Read the model definition and answer for the solid it produces. Units are mm, in the model's axes. A direction names the side the tool comes from. Coordinates: 2 decimals unless noted, no trailing zeros. Write each loop counter-clockwise with the first axis right and the second up, starting at its lowest first coordinate (ties: lowest second). Pieces come first, ordered by that corner, then holes. Notation, with made-up numbers: (15.25, 36.5) - (36.25, 36.5) arc R35 ccw to (36.25, 69.5) - close; hole circle Ø2 at (35, 27.5). An arc over 180 degrees is marked (long way). Use a Markdown table: item, result.
Autodesk Inventor part; units mm, degrees
ref_plane "YZ Plane" through (0, 0, 0) normal (1, 0, 0) x (0, 1, 0)
ref_plane "XZ Plane" through (0, 0, 0) normal (0, 1, 0) x (-1, 0, 0)
ref_plane "XY Plane" through (0, 0, 0) normal (0, 0, 1) x (1, 0, 0)
sketch "Sketch1" plane through (0, 0, 0) normal (0, 0, 1) x (1, 0, 0)
  line L0 (0, 0) -> (127, 0)
  line L1 (127, 0) -> (127, 50.8)
  line L2 (127, 50.8) -> (0, 50.8)
  line L3 (0, 50.8) -> (0, 0)
  line L4 (0, 25.4) -> (6.35, 25.4)
  line L5 (0, 25.4) -> (6.35, 25.4) construction
  line L6 (6.35, 25.4) -> (15.367, 25.4)
  line L7 (127, 25.4) -> (120.65, 25.4)
  line L8 (127, 25.4) -> (133.35, 25.4) construction
  line L9 (15.367, 25.4) -> (15.367, 34.417)
  line L10 (15.367, 25.4) -> (24.384, 25.4) construction
  line L11 (15.367, 25.4) -> (15.367, 16.383)
  line L12 (20.3793, 14.0457) -> (11.3996, 24.7474)
  line L13 (24.8663, 36.7543) -> (33.846, 26.0526) construction
  line L14 (11.3996, 24.7474) -> (25.2144, 36.3394)
  line L15 (25.2144, 36.3394) -> (34.1942, 25.6377)
  line L16 (15.367, 25.4) -> (11.049, 25.4)
  arc A0 (20.3793, 14.0457) -> (34.1942, 25.6377) centre (22.6228, 25.4) ccw
  line L17 (120.65, 25.4) -> (131.064, 25.4) construction
  line L18 (22.6228, 25.4) -> (107.7128, 25.4)
  line L19 (22.6228, 25.4) -> (107.7128, 25.4) construction
  line L20 (22.6228, 25.4) -> (87.3928, 25.4)
  line L21 (22.6228, 25.4) -> (87.3928, 25.4) construction
  line L22 (87.3928, 25.4) -> (107.7128, 25.4)
  line L23 (107.7128, 25.4) -> (87.3928, 25.4) construction
  line L24 (107.7128, 29.845) -> (87.3928, 29.845)
  line L25 (87.3928, 20.955) -> (107.7128, 20.955)
  arc A1 (107.7128, 20.955) -> (107.7128, 29.845) centre (107.7128, 25.4) ccw
  arc A2 (87.3928, 29.845) -> (87.3928, 20.955) centre (87.3928, 25.4) ccw
  line L26 (107.7128, 25.4) -> (107.7128, 35.814)
  line L27 (107.7128, 25.4) -> (118.1268, 25.4) construction
  line L28 (107.7128, 35.814) -> (118.1268, 35.814)
  line L29 (107.7128, 35.814) -> (118.1268, 35.814) construction
  line L30 (107.7128, 14.986) -> (118.1268, 14.986)
  line L31 (97.5528, 25.4) -> (97.5528, 27.2043)
  line L32 (87.3928, 35.814) -> (76.9788, 35.814)
  line L33 (87.3928, 35.814) -> (76.9788, 35.814) construction
  line L34 (87.3928, 14.986) -> (76.9788, 14.986)
  line L35 (97.5528, 35.814) -> (97.5528, 14.986)
  line L36 (97.5528, 35.814) -> (118.3808, 35.814) construction
  line L37 (118.1268, 35.814) -> (76.9788, 35.814) construction
  line L38 (118.1268, 37.846) -> (76.9788, 37.846)
  line L39 (76.9788, 33.782) -> (118.1268, 33.782)
  arc A3 (118.1268, 33.782) -> (118.1268, 37.846) centre (118.1268, 35.814) ccw
  arc A4 (76.9788, 37.846) -> (76.9788, 33.782) centre (76.9788, 35.814) ccw
  line L40 (118.1268, 14.986) -> (76.9788, 14.986) construction
  line L41 (118.1268, 17.018) -> (76.9788, 17.018)
  line L42 (76.9788, 12.954) -> (118.1268, 12.954)
  arc A5 (118.1268, 12.954) -> (118.1268, 17.018) centre (118.1268, 14.986) ccw
  arc A6 (76.9788, 17.018) -> (76.9788, 12.954) centre (76.9788, 14.986) ccw
  dimension "d1" = 127
  dimension "d2" = 50.8
  dimension "d3" = 6.35
  dimension "d4" = 0
  dimension "d5" = 9.017
  dimension "d6" = 180
  dimension "d7" = 6.35
  dimension "d8" = 180
  dimension "d11" = 9.017
  dimension "d12" = 90
  dimension "d13" = 13.97
  dimension "d14" = 180
  dimension "d15" = 4.318
  dimension "d18" = 85.09
  dimension "d20" = 64.77
  dimension "d22" = 8.89
  dimension "d23" = 10.414
  dimension "d24" = 90
  dimension "d25" = 10.414
  dimension "d26" = 0
  dimension "d27" = 90
  dimension "d28" = 4.064
  dimension "d29" = 4.064
  dimension "d41" = 20.828
extrude "Extrusion1" add sketch "Sketch1" along normal blind 12.7 contours L3 L2 L1 L0 | L35 L39 L26 L24
sketch "Sketch2" plane through (0, 0, 12.7) normal (0, 0, 1) x (1, 0, 0)
  line L0 (127, 0) -> (127, 50.8)
  line L1 (71.2806, 47.625) -> (123.825, 47.625)
  line L2 (123.825, 47.625) -> (123.825, 3.175)
  line L3 (123.825, 3.175) -> (71.2806, 3.175)
  line L4 (71.2806, 47.625) -> (71.2806, 3.175)
  line L5 (127, 50.8) -> (68.1056, 50.8)
  line L6 (68.1056, 0) -> (127, 0)
  line L7 (68.1056, 50.8) -> (68.1056, 0)
  point P0 (0, 0)
extrude "Extrusion2" cut sketch "Sketch2" against normal blind 6.096 contours L1 L2 L3 L4
fillet "Fillet1" radius 5.08 2 edges at (127, 0, 6.35) (127, 50.8, 6.35)
fillet "Fillet2" radius 3.175 4 edges at (123.825, 47.625, 9.652) (71.2806, 47.625, 9.652) (71.2806, 3.175, 9.652) (123.825, 3.175, 9.652)
sketch "Sketch3" plane through (0, 0, 12.7) normal (0, 0, 1) x (1, 0, 0)
  line L0 (121.92, 50.8) -> (0, 50.8)
  line L1 (60.96, 50.8) -> (60.96, -0.3735)
  line L2 (60.96, 50.8) -> (112.1335, 50.8) construction
  line L3 (60.96, -0.3735) -> (60.96, 12.3265)
  line L4 (60.96, 12.3265) -> (43.18, 12.3265)
  circle A0 centre (43.18, 12.3265) radius 2.286
  circle A1 centre (45.72, 38.1) radius 2.286
  line L5 (0, 50.8) -> (0, 0)
  line L6 (0, 25.4) -> (12.7, 25.4)
  line L7 (0, 25.4) -> (12.7, 25.4) construction
  line L8 (12.7, 25.4) -> (12.7, 8.89)
  line L9 (12.7, 25.4) -> (29.21, 25.4) construction
  circle A2 centre (12.7, 8.89) radius 2.286
  circle A3 centre (12.7, 41.91) radius 2.286
  line L10 (60.96, 25.2132) -> (58.42, 25.2132)
  line L11 (60.96, 25.2132) -> (63.5, 25.2132) construction
  line L12 (58.42, 25.2132) -> (58.42, 37.9132)
  circle A4 centre (58.42, 37.9132) radius 2.286
  circle A5 centre (58.42, 12.5132) radius 2.286
  point P0 (3.175, 50.8)
  point P1 (0, 47.625)
  point P2 (0, 3.175)
  dimension "d42" = 90
  dimension "d43" = 12.7
  dimension "d44" = 0
  dimension "d45" = 17.78
  dimension "d46" = 4.572
  dimension "d47" = 12.7
  dimension "d48" = 0
  dimension "d49" = 16.51
  dimension "d50" = 90
  dimension "d51" = 4.572
  dimension "d52" = 2.54
  dimension "d53" = 180
  dimension "d54" = 4.572
extrude "Extrusion3" cut sketch "Sketch3" against normal blind 25.4
fillet "Fillet3" radius 19.05 2 edges at (0, 50.8, 6.35) (0, 0, 6.35)
properties part number "Skateboard Motor Bracket"
(1) Each of these flat-tipped pins is pushed along its axis until it touches: P1, Ø4, axis at x = 89.5, y = 11, coming from the -Z side; P2, Ø4, axis at y = 34, z = 2.5, coming from the -X side; P3, Ø1.5, axis at x = 13.5, z = 6, coming from the -Y side. Where does it stop, or does it pass through?
Report:
| item | result |
|---|---|
| P1 | stops at z = 0 |
| P2 | stops at x = 0 |
| P3 | stops at y = 0.61 |
(2) A cutting plane is placed at A-A, the plane x = 58.42. Write down the section's boundary in (y, z).
Report:
| item | result |
|---|---|
| outline | (0, 0) - (10.23, 0) - (10.23, 12.7) - (0, 12.7) - close; (14.8, 0) - (35.63, 0) - (35.63, 12.7) - (14.8, 12.7) - close; (40.2, 0) - (50.8, 0) - (50.8, 12.7) - (40.2, 12.7) - close |
(3) A cutting plane is placed at C-C, the plane y = 41.91. Write down the section's boundary in (x, z) (1 decimal), and give its area (3 significant figures).
Report:
| item | result |
|---|---|
| outline | (2.9, 0) - (10.4, 0) - (10.4, 12.7) - (2.9, 12.7) - close; (15, 0) - (127, 0) - (127, 12.7) - (123.8, 12.7) - (123.8, 6.6) - (71.3, 6.6) - (71.3, 12.7) - (15, 12.7) - close |
| area | 1,200 mm² |
(4) A cutting plane is placed at B-B, the plane z = 10. Count the separate pieces of the cut face and the enclosed holes in it, and give its area (3 significant figures).
Report:
| item | result |
|---|---|
| separate pieces | 1 |
| enclosed holes | 8 |
| area | 3,550 mm² |
(5) For faces 1 (the cylindrical face through (74.947, 14.941, 3.256)), 2 (the flat face through (97, 47.625, 10)), 3 (the cylindrical face through (125.472, 1.449, 6.439)), determine the directions among +Z, -Z, +X, -X, +Y, -Y from which every point of the face is accessible in a straight line to the end or side of a thin tool.
Report:
| item | result |
|---|---|
| face 1 | +Z, -Z |
| face 2 | +Z |
| face 3 | +Z, -Z, +X, -Y |
(6) The mould has two halves that part along X. Classify faces 4 (the cylindrical face through (72.186, 46.67, 9.609)), 5 (the flat face through (0, 25, 6)), 6 (the flat face through (48, 26, 12.7)): pulls with the +X half, pulls with the -X half, needs draft (parallel to the pull), parting line crosses it, or undercut.
Report:
| item | result |
|---|---|
| face 4 | undercut |
| face 5 | pulls with the -X half |
| face 6 | needs draft |
(7) Straight lines are drawn through the part: L1, parallel to Y at x = 58.42, z = 5.5; L2, parallel to Y at x = 87.5, z = 4 (3 decimals); L3, parallel to Y at x = 119, z = 6.75 (3 decimals). For each, find the intervals that lie inside material, in ascending order.
Report:
| item | result |
|---|---|
| L1 | y = 0 to 10.23, 14.8 to 35.63, 40.2 to 50.8 |
| L2 | y = 0 to 12.954, 17.018 to 20.955, 29.845 to 33.782, 37.846 to 50.8 |
| L3 | y = 0 to 3.175, 47.625 to 50.8 |
